Source: CAD feature listing. Evaluate the final solid. Frame: model axes, mm. Face numbers are marked on the shaded views. Round coordinates to 2 decimals unless told otherwise and drop trailing zeros. Loops run counter-clockwise (first coordinate to the right, second up) from the corner with the lowest first, then second, coordinate; pieces in that order, holes last.
Item 1: Section query B-B on z = 12.5. Return loops of the section in (x, y).
Item 2: Section query A-A on z = 21.75. Return loops of the section in (x, y), then the cut area to 3 significant figures.
Item 3: Section query D-D on x = 7. Return loops of the section in (y, z).
Item 4: Ray query, L1, parallel to X at y = 29, z = 10; L2, parallel to Z at x = -22.5, y = -51; L3, parallel to X at y = 25.5, z = 15. Return the intervals inside material, ascending.
Item 5: Pull-direction query (X, two-part tool) for the marked faces 1, 2 and 3; classes: released by +X, released by -X, zero draft, split by the parting line, or undercut.
Item 6: First-contact query: P1, Ø15, axis at x = -2.5, y = -65, coming from the -Z side; P2, Ø4, axis at y = 22.58, z = 12.5, coming from the -X side; P3, Ø10.5, axis at y = 22.58, z = 12.5, coming from the +X side; P4, Ø1.1, axis at x = -5, z = 24.5, coming from the +Y side. Flat tips, straight axial feed; report the tip coordinate or a pass-through.
Item 7: Section query C-C on y = -3. Return loops of the section in (x, z), then the cut area to 3 significant figures.
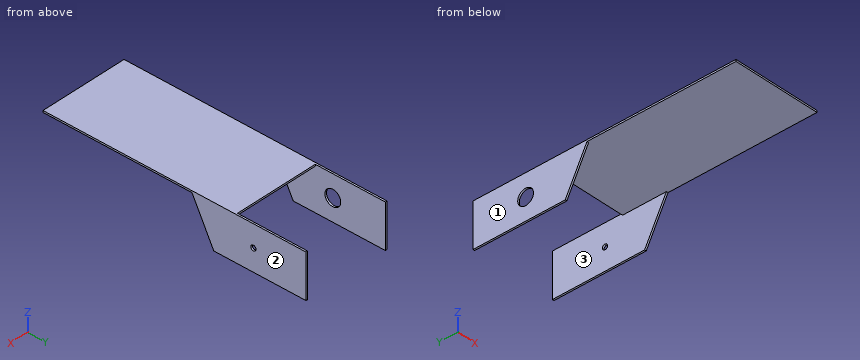
```python
from build123d import *

# Parameters (mm, degrees)
CROQUIS2_W              = 50
CROQUIS2_H              = 150
SALIENTE_EXTRUIR1_DEPTH = 25
CROQUIS6_W              = 48
CROQUIS6_H              = 40
CORTAR_EXTRUIR1_DEPTH   = 25
VACIADO2_START          = -31.864905155
VACIADO2_OUTLINE_W      = 110
VACIADO2_OUTLINE_H      = 23
VACIADO2_DEPTH          = 48
CROQUIS8_R              = 4.5
CORTAR_EXTRUIR3_DEPTH   = 1
CROQUIS9_W              = 48
CROQUIS9_H              = 110
CORTAR_EXTRUIR4_DEPTH   = 10
CORTAR_EXTRUIR5_DEPTH   = 1
CORTAR_EXTRUIR6_DEPTH   = 1
CROQUIS12_R             = 1.5
CORTAR_EXTRUIR7_DEPTH   = 1


# Read off the part's stored shape, not the designer's step: Vaciado2
with BuildPart() as part:
    # Croquis2 → Saliente-Extruir1 (new body)
    with BuildSketch(Plane.XY):
        with Locations((-7.864905155, -22.416151752)):
            Rectangle(CROQUIS2_W, CROQUIS2_H)
    extrude(amount=SALIENTE_EXTRUIR1_DEPTH)

    # Croquis6 → Cortar-Extruir1 (cut)
    with BuildSketch(Plane(origin=(0, 0, 0), x_dir=(-1, 0, 0), z_dir=(0, 0, -1))):
        with Locations((7.864905155, 32.583848248)):
            Rectangle(CROQUIS6_W, CROQUIS6_H)
    extrude(amount=-CORTAR_EXTRUIR1_DEPTH, mode=Mode.SUBTRACT)

    # Vaciado2 outline → Vaciado2 (cut)
    with BuildSketch(Plane.YZ.offset(VACIADO2_START)):
        with Locations((-42.416151752, 12.5)):
            Rectangle(VACIADO2_OUTLINE_W, VACIADO2_OUTLINE_H)
    extrude(amount=VACIADO2_DEPTH, mode=Mode.SUBTRACT)

    # Croquis8 → Cortar-Extruir3 (cut)
    with BuildSketch(Plane.ZY.offset(32.864905155)):
        with Locations(Location((12.5, 22.583848248, 0), (0, 0, 270))):
            Circle(CROQUIS8_R)
    extrude(amount=-CORTAR_EXTRUIR3_DEPTH, mode=Mode.SUBTRACT)

    # Croquis9 → Cortar-Extruir4 (cut)
    with BuildSketch(Plane(origin=(0, 0, 0), x_dir=(-1, 0, 0), z_dir=(0, 0, -1))):
        with Locations((7.864905155, -42.416151752)):
            Rectangle(CROQUIS9_W, CROQUIS9_H)
    extrude(amount=-CORTAR_EXTRUIR4_DEPTH, mode=Mode.SUBTRACT)

    # Croquis10 → Cortar-Extruir5 (cut)
    with BuildSketch(Plane.ZY.offset(32.864905155)):
        Polygon((0, 0), (24, -12.416151752), (24, -97.416151752), (0, -97.416151752), align=None)
    extrude(amount=-CORTAR_EXTRUIR5_DEPTH, mode=Mode.SUBTRACT)

    # Croquis11 → Cortar-Extruir6 (cut)
    with BuildSketch(Plane(origin=(17.135094845, 0, 0), x_dir=(0, 0, -1), z_dir=(1, 0, 0))):
        Polygon((0, 0), (-24, -12.416151752), (-24, -97.416151752), (0, -97.416151752), align=None)
    extrude(amount=-CORTAR_EXTRUIR6_DEPTH, mode=Mode.SUBTRACT)

    # Croquis12 → Cortar-Extruir7 (cut)
    with BuildSketch(Plane(origin=(17.135094845, 0, 0), x_dir=(0, 0, -1), z_dir=(1, 0, 0))):
        with Locations(Location((-12.5, 22.583848248, 0), (0, 0, 90))):
            Circle(CROQUIS12_R)
    extrude(amount=-CORTAR_EXTRUIR7_DEPTH, mode=Mode.SUBTRACT)


solid = part.part
```
Data:
1. outline: (-32.86, -6.47) - (-31.86, -6.47) - (-31.86, 18.08) - (-32.86, 18.08) - close; (-32.86, 27.08) - (-31.86, 27.08) - (-31.86, 52.58) - (-32.86, 52.58) - close; (16.14, -6.47) - (17.14, -6.47) - (17.14, 21.08) - (16.14, 21.08) - close; (16.14, 24.08) - (17.14, 24.08) - (17.14, 52.58) - (16.14, 52.58) - close
2. outline: (-32.86, -11.25) - (-31.86, -11.25) - (-31.86, 52.58) - (-32.86, 52.58) - close; (16.14, -11.25) - (17.14, -11.25) - (17.14, 52.58) - (16.14, 52.58) - close
2. area: 128 mm2
3. outline: (-97.42, 24) - (12.58, 24) - (12.58, 25) - (-97.42, 25) - close
4. L1: x = -32.86 to -31.86, 16.14 to 17.14
4. L2: z = 24 to 25
4. L3: x = 16.14 to 17.14
5. face 1: released by -X
5. face 2: released by +X
5. face 3: undercut
6. P1: stops at z = 24
6. P2: stops at x = 16.14
6. P3: stops at x = 17.14
6. P4: stops at y = 12.58
7. outline: (-32.86, 5.8) - (-31.86, 5.8) - (-31.86, 24) - (16.14, 24) - (16.14, 5.8) - (17.14, 5.8) - (17.14, 25) - (-32.86, 25) - close
7. area: 86.4 mm2
